Autodesk Inventor part; units mm, degrees
ref_plane "YZ Plane" through (0, 0, 0) normal (1, 0, 0) x (0, 1, 0)
ref_plane "XZ Plane" through (0, 0, 0) normal (0, 1, 0) x (-1, 0, 0)
ref_plane "XY Plane" through (0, 0, 0) normal (0, 0, 1) x (1, 0, 0)
sketch "Sketch1" plane through (0, 0, 0) normal (0, 0, 1) x (1, 0, 0)
  line L0 (-14.822, 23.7423) -> (29.878, 23.7423)
  line L1 (29.878, 23.7423) -> (29.878, -7.2577)
  line L2 (29.878, -7.2577) -> (-14.822, -7.2577)
  line L3 (-14.822, -7.2577) -> (-14.822, 23.7423)
  line L4 (31.278, 25.1423) -> (-16.222, 25.1423)
  line L5 (-16.222, 25.1423) -> (-16.222, -8.6577)
  line L6 (-16.222, -8.6577) -> (31.278, -8.6577)
  line L7 (31.278, -8.6577) -> (31.278, 25.1423)
  point P0 (0, 0)
  dimension "d0" = 44.7
  dimension "d1" = 31
  dimension "d2" = 1.4
extrude "Extrusion1" add sketch "Sketch1" along normal blind 17
sketch "Sketch2" plane through (0, 0, 17) normal (0, 0, 1) x (1, 0, 0)
  line L0 (31.278, 25.1423) -> (-16.222, 25.1423)
  line L1 (-16.222, 25.1423) -> (-16.222, -8.6577)
  line L2 (-16.222, -8.6577) -> (31.278, -8.6577)
  line L3 (31.278, -8.6577) -> (31.278, 25.1423)
  point P0 (0, 0)
extrude "Extrusion2" add sketch "Sketch2" along normal blind 1.4
sketch "Sketch4" plane through (0, 0, 17) normal (0, 0, -1) x (-1, 0, 0)
  circle A0 centre (-6.628, 9.5599) radius 12.6
  line L0 (-29.878, -7.2577) -> (-29.878, 23.7423)
  line L1 (14.822, 23.7423) -> (14.822, -7.2577)
  point P0 (0, 0)
  dimension "d7" = 23.25
  dimension "d8" = 44.7
  dimension "d9" = 25.2
extrude "Extrusion3" cut sketch "Sketch4" against normal blind 1.4
sketch "Sketch5" plane through (0, 0, 17) normal (0, 0, -1) x (-1, 0, 0)
  circle A0 centre (-6.628, 9.5599) radius 12.6
  circle A1 centre (-6.628, 9.5599) radius 14
  point P0 (0, 0)
  dimension "d12" = 1.4
extrude "Extrusion4" add sketch "Sketch5" along normal blind 2.2
chamfer "Chamfer1" distance 1 angle 45 1 edges at (20.628, 9.5599, 17)
sketch "Sketch6" plane through (0, 0, 0) normal (0, 0, -1) x (-1, 0, 0)
  line L0 (16.222, 25.1423) -> (16.222, -8.6577)
  line L1 (16.222, -8.6577) -> (-31.278, -8.6577)
  line L2 (-31.278, -8.6577) -> (-31.278, 25.1423)
  line L3 (14.822, 23.7423) -> (14.822, -7.2577)
  line L4 (14.822, -7.2577) -> (-29.878, -7.2577)
  line L5 (-29.878, -7.2577) -> (-29.878, 23.7423)
  line L6 (14.822, 23.7423) -> (-1.7434, 23.7423)
  line L7 (14.822, 23.7423) -> (14.822, 25.1423)
  line L8 (14.822, 25.1423) -> (16.222, 25.1423)
  line L9 (-29.878, 23.7423) -> (-29.878, 25.1423)
  line L10 (-29.878, 25.1423) -> (-31.278, 25.1423)
  point P0 (0, 0)
extrude "Extrusion5" add sketch "Sketch6" along normal blind 2
sketch "Sketch8" plane through (0, 0, -2) normal (0, 0, -1) x (-1, 0, 0)
  line L0 (14.822, -7.2577) -> (14.822, 23.7423)
  line L1 (-29.878, 23.7423) -> (-29.878, -7.2577)
  line L2 (14.822, -7.2577) -> (-29.878, -7.2577)
  line L3 (-29.878, -7.2577) -> (-29.878, 23.7423)
  line L4 (14.822, 23.7423) -> (14.822, -7.2577)
  line L5 (-29.678, -7.0577) -> (14.622, -7.0577)
  line L6 (14.622, -7.0577) -> (14.622, 23.5423)
  line L7 (-29.678, 23.5423) -> (-29.678, -7.0577)
  line L8 (14.622, 23.5423) -> (14.622, 23.7423)
  line L9 (-29.678, 23.5423) -> (-29.678, 23.7423)
  line L10 (-29.878, 23.7423) -> (14.822, 23.7423)
  line L11 (-29.878, 23.7423) -> (-29.678, 23.7423)
  line L12 (14.622, 23.7423) -> (14.822, 23.7423)
  point P0 (0, 0)
  dimension "d24" = 0.2
extrude "Extrusion7" add sketch "Sketch8" against normal blind 0.4 contours L2 L1 L10 L9 L7 L5 L6 L8 L0
chamfer "Chamfer2" distance 0.2 angle 45 3 edges at (7.528, -7.0577, -1.6) (-14.622, 8.3423, -1.6) (29.678, 8.3423, -1.6)
chamfer "Chamfer3" distance 2 angle 45 1 edges at (-14.822, 23.7423, 8.5)
chamfer "Chamfer4" distance 2 angle 45 1 edges at (29.878, 23.7423, 8.5)
sketch "Sketch9" plane through (-14.822, 25.1423, 0) normal (0, 1, 0) x (1, 0, 0)
  line L0 (42.7, 0) -> (2, 0)
  line L1 (31.7, 0) -> (11, 0)
  line L2 (11, 0) -> (11, -1.2)
  line L3 (11, -1.2) -> (31.7, -1.2)
  line L4 (31.7, -1.2) -> (31.7, 0)
  line L5 (44.7, 0) -> (44.7, -17)
  line L6 (0, -17) -> (0, 0)
  point P0 (14.822, 0)
  dimension "d48" = 13
  dimension "d49" = 11
  dimension "d50" = 1.2
extrude "Extrusion8" cut sketch "Sketch9" against normal up to surface (1.4 mm away)
fillet "Fillet3" radius 2 8 edges at (7.528, 25.1423, 18.4) (-16.222, 8.2423, 18.4) (-16.222, 25.1423, 8.2) (-16.222, -8.6577, 8.2) (7.528, -8.6577, 18.4) (31.278, 8.2423, 18.4) (31.278, -8.6577, 8.2) (31.278, 25.1423, 8.2)
properties part number "lupa-card-c-mount"
Input: part model. Units: mm. Frame: model coordinates. A direction names the side the tool comes from. Coordinates: 2 decimals unless noted, no trailing zeros. Loops run counter-clockwise (first coordinate to the right, second up) from the corner with the lowest first, then second, coordinate; pieces in that order, holes last. Notation, with made-up numbers: (36.5, 36) -> (47.5, 36) arc R24 cw to (47.5, 62) -> close; hole circle Ø3 at (-6.5, 6.5). An arc over 180 degrees is marked (long way). Write each question's results on one line, items separated by ' | '. Start each with the question number.
Q1. Pin query (flat end, axial travel): pin 1 (1.7 mm diameter, centred on x = 25.5, y = 24, fed in from -Z); pin 2 (15.5 mm diameter, centred on x = 3, y = 3.5, fed in from -Z); pin 3 (0.7 mm diameter, centred on x = 6, y = 24.5, fed in from -Z). Return the tip coordinate at first contact, or that it passes through.
Q2. Reachability of faces 1 (the flat face through (8, -7.258, 8)), 2 (the flat face through (17, 17, 14.8)), 3 (the cylindrical face through (-15.62, 24.57, 7.33)), 4 (the flat face through (-3.822, 24, 1)) from +Z, -Z, +X, -X, +Y, -Y: full face, straight path, thin tool, end or side. Return the list, or none.
Q3. Section A-A, the plane z = 6.5. Return the cut outline in (x, y).
Q4. Ray query, line 1 (Y direction, x = 21.5, z = 11.25); line 2 (X direction, y = 11.5, z = 4); line 3 (Y direction, x = 19.5, z = 15.25). Return the intervals inside material, ascending. Write a range as from..to.
Q5. Pull-direction query (Y, two-part tool) for faces 5 (the flat face through (-16.222, 8, 7)), 6 (the cylindrical face through (-0.898, -2.245, 15.408)), 7 (the cylindrical face through (7.833, -8.056, 17.83)); classes: released by +Y, released by -Y, zero draft, split by the parting line, or undercut.
Found:
1) pin 1: z = 0 | pin 2: z = 14.8 | pin 3: z = 1.2
2) face 1: none | face 2: -Z | face 3: +Z, -Z, -X, +Y | face 4: -Z, +Y
3) outline: (-16.22, -6.66) arc R2 ccw to (-14.22, -8.66) -> (29.28, -8.66) arc R2 ccw to (31.28, -6.66) -> (31.28, 23.14) arc R2 ccw to (29.28, 25.14) -> (-14.22, 25.14) arc R2 ccw to (-16.22, 23.14) -> close; hole (-14.82, -7.26) -> (29.88, -7.26) -> (29.88, 21.74) -> (27.88, 23.74) -> (-12.82, 23.74) -> (-14.82, 21.74) -> close
4) line 1: -8.66..-7.26, 23.74..25.14 | line 2: -16.22..-14.82, 29.88..31.28 | line 3: -8.66..-7.26, 4.05..15.07, 23.74..25.14
5) face 5: zero draft | face 6: undercut | face 7: released by -Y
